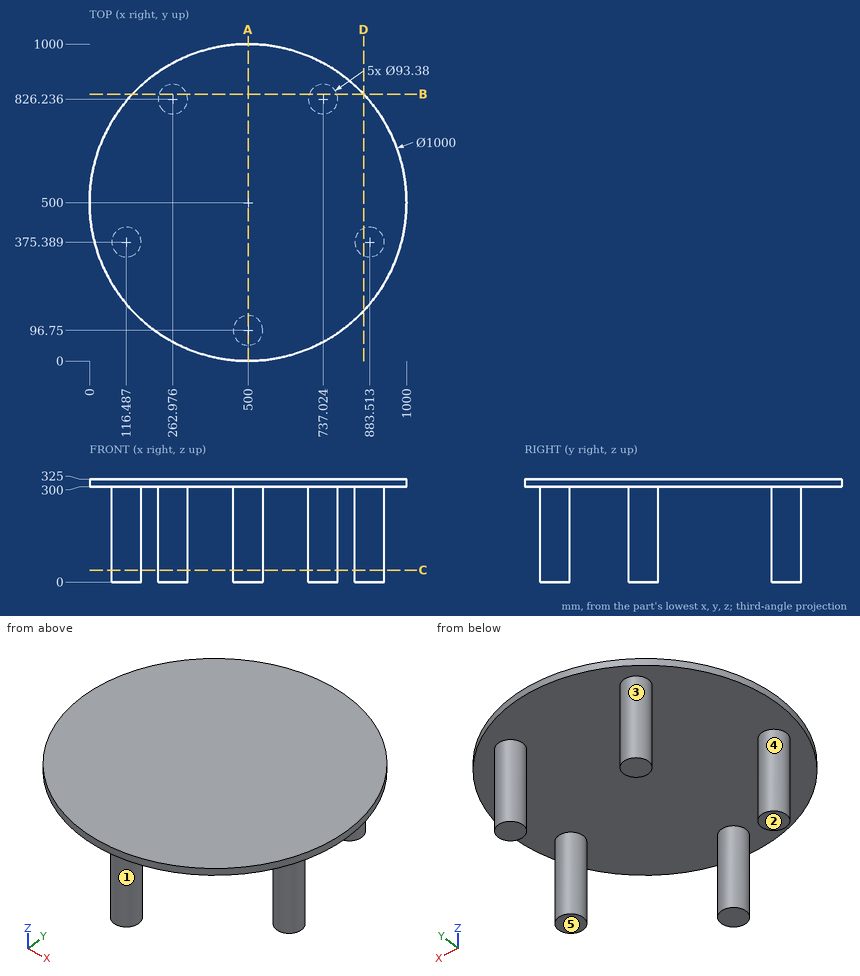
Could you check a few things on this drawing? It's one solid part, dimensions in mm from its lowest x, y, z. A direction names the side the tool comes from. Give positions to 0.01 mm unless a question says otherwise; leave off trailing zeros. Order: outer loops, then holes, each group sorted by start corner. A loop starts at its lowest first (then second) coordinate and runs counter-clockwise, first axis right, second up. Notation, with made-up numbers: (-2.75, 61.5) - (35.25, 61.5) arc R32 ccw to (35.25, 93.5) - close; hole circle Ø2 at (-39.5, -25). An arc over 180 degrees is marked (long way). One line per question, with ' | ' between items. Start each with the question number.
Item 1: For the marked faces 4 and 5, which set-ups out of +Z, -Z, +X, -X, +Y, -Y let a thin tool reach every point of the face, with its end or its side?
Item 2: I want a section at D-D on x = 864.5. Write out the boundary of the cut face in (y, z) (1 decimal), then the cut area to 3 significant figures.
Item 3: Thinking about a two-plate mould opening in X: for the marked faces 1, 2 and 3, which applies, pulls with the +X half, pulls with the -X half, needs draft (parallel to the pull), parting line crosses it, or undercut?
Item 4: I need wall thicknesses on probe 1 along X at (y, z) = (798.5, 19.5) (1 decimal); probe 2 along Z at (x, y) = (273, 486); probe 3 along X at (y, z) = (624.5, 308). Which ranges of each line are inside material? Lowest first, please. Write a range as [from, to].
Item 5: I want a section at A-A on x = 500. Write out the boundary of the cut face in (y, z), then the cut area to 3 significant figures.
Item 6: I want a section at C-C on z = 37.5. Give the number of separate pieces and of enclosed holes in the cut face, then the cut area to 3 significant figures.
Item 7: I want a section at B-B on y = 842. Write out the boundary of the cut face in (x, z), then the cut area to 3 significant figures.
Item 8: I'm going to push flat-ended pins straight in: pin 1 Ø1.5 at (y, z) = (413.5, 145.5) entering from +X (1 decimal); pin 2 Ø3 at (x, y) = (815, 386.5) entering from -Z; pin 3 Ø4 at (x, z) = (746, 286.5) entering from +Y. Where does each tip first touch, or does it pass through?
Verdict:
1) face 4: -Z | face 5: -Z, +X, -X, +Y, -Y
2) outline: (157.7, 300) - (332.7, 300) - (332.7, 0) - (418, 0) - (418, 300) - (842.3, 300) - (842.3, 325) - (157.7, 325) - close | area: 42,700 mm^2
3) face 1: parting line crosses it | face 2: needs draft | face 3: undercut
4) probe 1: [225.4, 300.5], [699.5, 774.6] | probe 2: [300, 325] | probe 3: [15.75, 984.25]
5) outline: (0, 300) - (50.06, 300) - (50.06, 0) - (143.44, 0) - (143.44, 300) - (1000, 300) - (1000, 325) - (0, 325) - close | area: 53,000 mm^2
6) separate pieces: 5 | enclosed holes: 0 | area: 34,200 mm^2
7) outline: (135.26, 300) - (219.03, 300) - (219.03, 0) - (306.92, 0) - (306.92, 300) - (693.08, 300) - (693.08, 0) - (780.97, 0) - (780.97, 300) - (864.74, 300) - (864.74, 325) - (135.26, 325) - close | area: 71,000 mm^2
8) pin 1: x = 911.5 | pin 2: z = 300 | pin 3: y = 872.4
